from build123d import *

# Parameters (mm, degrees)
SKETCH1_W               = 20
SKETCH1_H               = 11.5
BOSS_EXTRUDE1_DEPTH     = 5
SKETCH2_W               = 5
SKETCH2_H               = 11.5
BOSS_EXTRUDE2_DEPTH     = 25
SKETCH3_W               = 18
SKETCH3_H               = 11.75
BOSS_EXTRUDE3_DEPTH     = 5
CUT_EXTRUDE1_DEPTH      = 5
CUT_EXTRUDE2_DEPTH      = 33.186953879
CUT_EXTRUDE2_DEPTH_BACK = 33.186953879
SKETCH5_R               = 2
FILLET1_R               = 9
FILLET7_R               = 5
FILLET8_R               = 1
FILLET9_R               = 2
CUT_EXTRUDE4_DEPTH      = 39.173943993
CUT_EXTRUDE4_DEPTH_BACK = 39.173943993
SKETCH10_R              = 1.5
SKETCH10_4_R            = 3.5
SKETCH10_4_R_2          = 1.5
BOSS_EXTRUDE7_DEPTH     = 11.5
FILLET13_R              = 1
FILLET16_R              = 5
SKETCH11_W              = 10
SKETCH11_H              = 2.875
BOSS_EXTRUDE8_DEPTH     = 7
CUT_EXTRUDE5_DEPTH      = 46.508927696
CUT_EXTRUDE5_DEPTH_BACK = 46.508927696
SKETCH12_R              = 2
FILLET17_R              = 3
FILLET18_R              = 3
FILLET19_R              = 3


with BuildPart() as part:
    # Sketch1 → Boss-Extrude1 (new body)
    with BuildSketch(Plane.XY):
        Rectangle(SKETCH1_W, SKETCH1_H)
    extrude(amount=BOSS_EXTRUDE1_DEPTH)

    # Sketch2 → Boss-Extrude2 (add)
    with BuildSketch(Plane.XY.offset(5)):
        with Locations((-7.5, 0)):
            Rectangle(SKETCH2_W, SKETCH2_H)
    extrude(amount=BOSS_EXTRUDE2_DEPTH)

    # Sketch3 → Boss-Extrude3 (add)
    with BuildSketch(Plane.XY.offset(30)):
        with Locations((-1, -0.125)):
            Rectangle(SKETCH3_W, SKETCH3_H)
    extrude(amount=BOSS_EXTRUDE3_DEPTH)

    # Sketch4 → Cut-Extrude1 (cut)
    with BuildSketch(Plane.ZY.offset(10)):
        with BuildLine():
            Line((15, 2.875), (25, 2.875))
            ThreePointArc((25, 2.875), (28, -0.125), (25, -3.125))
            Line((25, -3.125), (15, -3.125))
            ThreePointArc((15, -3.125), (12, -0.125), (15, 2.875))
        make_face()
    extrude(amount=-CUT_EXTRUDE1_DEPTH, mode=Mode.SUBTRACT)

    # Sketch5 → Cut-Extrude2 (cut, two sides: drawn at the far end of the back side and taken through both)
    with BuildSketch(Plane(origin=(0, 0, 30), x_dir=(-1, 0, 0), z_dir=(0, 0, -1)).offset(-CUT_EXTRUDE2_DEPTH_BACK)):
        with Locations((-2, -0.125)):
            Circle(SKETCH5_R)
    extrude(amount=CUT_EXTRUDE2_DEPTH + CUT_EXTRUDE2_DEPTH_BACK, mode=Mode.SUBTRACT)

    # Fillet1
    fillet1_edges = [part.edges().sort_by_distance(p)[0] for p in [
        (-10, 0, 0),
    ]]
    fillet(fillet1_edges, radius=FILLET1_R)

    # Fillet7
    fillet7_edges = [part.edges().sort_by_distance(p)[0] for p in [
        (8, -6, 32.5),
        (8, 5.75, 32.5),
    ]]
    fillet(fillet7_edges, radius=FILLET7_R)

    # Fillet8
    fillet8_edges = [part.edges().sort_by_distance(p)[0] for p in [
        (-10, -0.125, 12),
        (-10, -3.125, 20),
        (-10, -0.125, 28),
        (-10, 2.875, 20),
    ]]
    fillet(fillet8_edges, radius=FILLET8_R)

    # Fillet9
    fillet9_edges = [part.edges().sort_by_distance(p)[0] for p in [
        (-5, -0.125, 12),
        (-5, 2.875, 20),
        (-5, -0.125, 28),
        (-5, -3.125, 20),
    ]]
    fillet(fillet9_edges, radius=FILLET9_R - 0.0001)  # a hair under: the kernel refuses the full size

    # Sketch10 → Cut-Extrude4 (cut, two sides: drawn at the far end of the back side and taken through both)
    with BuildSketch(Plane.XZ.offset(5.75).offset(-CUT_EXTRUDE4_DEPTH_BACK)):
        with Locations((9, 2.5)):
            Circle(SKETCH10_R)
    extrude(amount=CUT_EXTRUDE4_DEPTH + CUT_EXTRUDE4_DEPTH_BACK, mode=Mode.SUBTRACT)

    # Sketch10<4> → Boss-Extrude7 (add)
    with BuildSketch(Plane.XZ.offset(5.75)):
        with Locations((9, 2.5)):
            Circle(SKETCH10_4_R)
        with Locations(Location((9, 2.5, 0), (0, 0, 270))):
            Circle(SKETCH10_4_R_2, mode=Mode.SUBTRACT)
    extrude(amount=-BOSS_EXTRUDE7_DEPTH)

    # Fillet13
    fillet13_edges = [part.edges().sort_by_distance(p)[0] for p in [
        (6.550510257, 0, 0),
        (6.550510257, 0, 5),
    ]]
    fillet(fillet13_edges, radius=FILLET13_R)

    # Fillet16
    fillet16_edges = [part.edges().sort_by_distance(p)[0] for p in [
        (-5, 0, 5),
    ]]
    fillet(fillet16_edges, radius=FILLET16_R - 0.0001)  # a hair under: the kernel refuses the full size

    # Sketch11 → Boss-Extrude8 (add)
    with BuildSketch(Plane.XY.offset(35)):
        with Locations((-8, 4.3125)):
            Rectangle(SKETCH11_W, SKETCH11_H)
        with Locations((-8, -4.5625)):
            Rectangle(SKETCH11_W, SKETCH11_H)
    extrude(amount=BOSS_EXTRUDE8_DEPTH)

    # Sketch12 → Cut-Extrude5 (cut, two sides: drawn at the far end of the back side and taken through both)
    with BuildSketch(Plane(origin=(0, 5.75, 0), x_dir=(1, 0, 0), z_dir=(0, 1, 0)).offset(-CUT_EXTRUDE5_DEPTH_BACK)):
        with Locations(Location((-9, -38, 0), (0, 0, 90))):
            Circle(SKETCH12_R)
    extrude(amount=CUT_EXTRUDE5_DEPTH + CUT_EXTRUDE5_DEPTH_BACK, mode=Mode.SUBTRACT)

    # Fillet17
    fillet17_edges = [part.edges().sort_by_distance(p)[0] for p in [
        (-10, -4.5625, 35),
        (-3, 4.3125, 35),
        (-3, -4.5625, 35),
        (-10, 4.3125, 35),
    ]]
    fillet(fillet17_edges, radius=FILLET17_R - 0.0001)  # a hair under: the kernel refuses the full size
    fillet17_2_edges = [part.edges().sort_by_distance(p)[0] for p in [
        (-13, 4.3125, 42),
        (-3, 4.3125, 42),
        (-3, -4.5625, 42),
        (-13, -4.5625, 42),
    ]]
    fillet(fillet17_2_edges, radius=FILLET17_R)

    # Fillet18
    fillet18_edges = [part.edges().sort_by_distance(p)[0] for p in [
        (-13, 4.3125, 35),
        (-13, -4.5625, 35),
    ]]
    fillet(fillet18_edges, radius=FILLET18_R)

    # Fillet19
    fillet19_edges = [part.edges().sort_by_distance(p)[0] for p in [
        (-10, -0.125, 35),
    ]]
    fillet(fillet19_edges, radius=FILLET19_R - 0.0001)  # a hair under: the kernel refuses the full size


solid = part.part
Geometry check sheet. Reference: the model listing, model coordinates, mm. A direction names the side the tool comes from. Coordinates: 2 decimals unless noted, no trailing zeros. Order: outer loops, then holes, each group sorted by start corner. A loop starts at its lowest first (then second) coordinate and runs counter-clockwise, first axis right, second up. Notation, with made-up numbers: (0, 13.25) -> (4, 13.25) arc R15 ccw to (4, 41.25) -> close; hole circle Ø2 at (-30.75, 88.5). An arc over 180 degrees is marked (long way). Use a Markdown table: item, result. Add a question column.
1. Cross-section at D-D (y = -1.5). Give the number of separate pieces and of enclosed holes in the cut face, and give its area (3 significant figures).
2. Mould release check, pull along X, two halves, no side actions. Record for faces 1 (the face through (-5, -6, 35)), 2 (the face through (7.67, -0.08, 1.81)), 3 (the face through (-13, 4, 38)): pulls with the +X half, pulls with the -X half, needs draft (parallel to the pull), parting line crosses it, or undercut.
3. Cross-section at A-A (x = 2). Enter the section's corners in (y, z) (3 decimals).
4. Go/stop test with flat-tipped pins: pin 1 Ø4 at (y, z) = (-2, 22) entering from -X; pin 2 Ø2 at (x, y) = (6.5, -3.5) entering from +Z; pin 3 Ø1.4 at (y, z) = (0, 33) entering from +X. Record where each tip stops, or that it passes through.
5. Set-up check for faces 4 (the face through (-5.5, -5.75, 10)), 5 (the face through (-8, -0.2, 12)), 6 (the face through (-3, -4.6, 38.5)): record each of +Z, -Z, +X, -X, +Y, -Y from which the full face is reachable in a straight line by a thin tool's end or side.
6. Material ranges on L1, parallel to Z at x = 5.5, y = 2.5; L2, parallel to Z at x = 9, y = 2.25; L3, parallel to X at y = 5.05, z = 38, recorded low to high.
7. Cross-section at C-C (x = 9). Enter the section's corners in (y, z).
8. Cross-section at B-B (z = 2.5). Enter the section's corners in (x, y) (3 decimals), and give its area (3 significant figures).
Filled sheet:
| question | item | result |
|---|---|---|
| 1 | separate pieces | 4 |
| 1 | enclosed holes | 1 |
| 1 | area | 203 mm2 |
| 2 | face 1 | needs draft |
| 2 | face 2 | undercut |
| 2 | face 3 | pulls with the -X half |
| 3 | outline | (-6, 30) -> (-2.125, 30) -> (-2.125, 35) -> (-6, 35) -> close; (-5.75, 0) -> (-2.125, 0) -> (-2.125, 5) -> (-5.75, 5) -> close; (1.875, 0) -> (5.75, 0) -> (5.75, 5) -> (1.875, 5) -> close; (1.875, 30) -> (5.75, 30) -> (5.75, 35) -> (1.875, 35) -> close |
| 4 | pin 1 | x = -9.99 |
| 4 | pin 2 | z = 35 |
| 4 | pin 3 | x = 8 |
| 5 | face 4 | -Z, +X, -X, -Y |
| 5 | face 5 | +X, -X |
| 5 | face 6 | +Z, +X, +Y, -Y |
| 6 | L1 | 0 to 5, 30 to 35 |
| 6 | L2 | -1 to 1, 4 to 6 |
| 6 | L3 | -13 to -11, -7 to -3 |
| 7 | outline | (-5.75, -1) -> (5.75, -1) -> (5.75, 1) -> (-5.75, 1) -> close; (-5.75, 4) -> (5.75, 4) -> (5.75, 6) -> (-5.75, 6) -> close |
| 8 | outline | (-7.225, -5.75) -> (7.5, -5.75) -> (7.5, 5.75) -> (-7.225, 5.75) -> close; (10.5, -5.75) -> (12.5, -5.75) -> (12.5, 5.75) -> (10.5, 5.75) -> close; hole circle Ø4 at (2, -0.125) |
| 8 | area | 180 mm2 |
